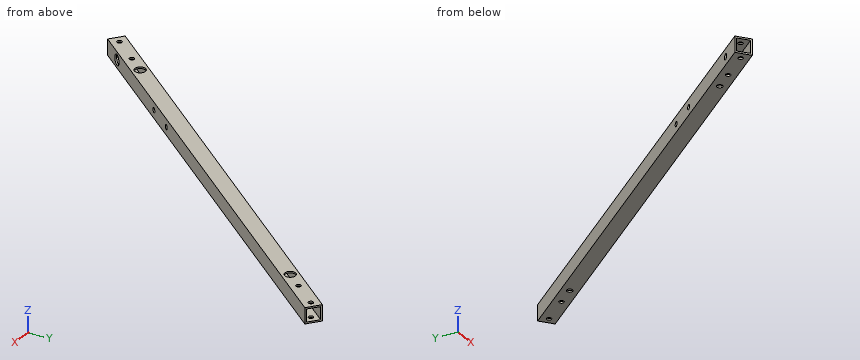
```python
from build123d import *

# Parameters (mm, degrees)
EXTRUDE_1_DEPTH             = 15
SHELL_1_T                   = -1.5
SKETCH_3_R                  = 2.25
SKETCH_3_R_2                = 2.7
CUT_EXTRUDE_1_DEPTH         = 25
SKETCH_5_R                  = 2.25
SKETCH_5_R_2                = 2.7
CUT_EXTRUDE_3_DEPTH         = 20
SKETCH_7_W                  = 15
SKETCH_7_H                  = 15
SKETCH_7_W_2                = 12
SKETCH_7_H_2                = 12
CUT_EXTRUDE_4_DEPTH         = 1
HOLE_WIZARD_10_0_10_1_D     = 10
HOLE_WIZARD_10_0_10_1_DEPTH = 1.5
HOLE_WIZARD_10_0_10_2_D     = 10
HOLE_WIZARD_10_0_10_2_DEPTH = 1.5


with BuildPart() as part:
    # ｽｹｯﾁ1 → ﾎﾞｽ - 押し出し1 (new body)
    with BuildSketch(Plane.XY):
        Polygon((306.8847856, 365.731045751), (0, 0), (-11.490666647, 9.641814145), (295.394118953, 375.372859896), align=None)
    extrude(amount=EXTRUDE_1_DEPTH)

    # ｼｪﾙ1
    shell_1_openings = [part.faces().sort_by_distance(p)[0] for p in [
        (301.139452276, 370.551952824, 7.5),
        (-5.745333323, 4.820907073, 7.5),
    ]]
    offset(amount=SHELL_1_T, openings=shell_1_openings, kind=Kind.INTERSECTION)

    # ｽｹｯﾁ3 → ｶｯﾄ - 押し出し1 (cut)
    with BuildSketch(Plane.XY.offset(15)):
        with Locations((-0.924426251, 10.566240396)):
            Circle(SKETCH_3_R)
        with Locations((18.35920204, 33.54757369)):
            Circle(SKETCH_3_R)
        with Locations((277.034916913, 341.825286207)):
            Circle(SKETCH_3_R)
        with Locations((296.318545204, 364.8066195)):
            Circle(SKETCH_3_R)
        with Locations((31.214954234, 48.868462552)):
            Circle(SKETCH_3_R_2)
        with Locations((264.179164719, 326.504397344)):
            Circle(SKETCH_3_R_2)
    extrude(amount=-CUT_EXTRUDE_1_DEPTH, mode=Mode.SUBTRACT)

    # ｽｹｯﾁ5 → ｶｯﾄ - 押し出し3 (cut)
    with BuildSketch(Plane(origin=(-11.490666647, 9.641814145, 0), x_dir=(0, 0, 1), z_dir=(-0.766044443, 0.64278761, 0))):
        with Locations((7.5, 141.822406051)):
            Circle(SKETCH_5_R)
        with Locations((7.5, 111.822406051)):
            Circle(SKETCH_5_R)
        with Locations((7.5, 22.5)):
            Circle(SKETCH_5_R_2)
    extrude(amount=-CUT_EXTRUDE_3_DEPTH, mode=Mode.SUBTRACT)

    # ｽｹｯﾁ7 → ｶｯﾄ - 押し出し4 (cut)
    with BuildSketch(Plane(origin=(306.8847856, 365.731045751, 0), x_dir=(0.766044443, -0.64278761, 0), z_dir=(0.64278761, 0.766044443, 0))):
        with Locations((-7.5, -7.5)):
            Rectangle(SKETCH_7_W, SKETCH_7_H)
        with Locations((-7.5, -7.5)):
            Rectangle(SKETCH_7_W_2, SKETCH_7_H_2, mode=Mode.SUBTRACT)
    extrude(amount=-CUT_EXTRUDE_4_DEPTH, mode=Mode.SUBTRACT)

    # Ø10.0 (10) 直径の穴1
    with Locations(Plane(origin=(0, 0, 0), x_dir=(0, 0, -1), z_dir=(0.766044443, -0.64278761, 0))):
        with Locations((-7.5, 22.5)):
            Hole(HOLE_WIZARD_10_0_10_1_D / 2, depth=HOLE_WIZARD_10_0_10_1_DEPTH)

    # Ø10.0 (10) 直径の穴2
    with Locations(Plane.XY.offset(15)):
        with Locations((31.214954234, 48.868462552), (264.179164719, 326.504397344)):
            Hole(HOLE_WIZARD_10_0_10_2_D / 2, depth=HOLE_WIZARD_10_0_10_2_DEPTH)


solid = part.part
```
Geometry check sheet. Reference: the model listing, model coordinates, mm. Give positions to 0.01 mm unless a question says otherwise; leave off trailing zeros. Order: outer loops, then holes, each group sorted by start corner. A loop starts at its lowest first (then second) coordinate and runs counter-clockwise, first axis right, second up. Notation, with made-up numbers: (33, -8) - (63, -8) arc R34 ccw to (63, 30) - close; hole circle Ø7 at (0.5, 71.5). An arc over 180 degrees is marked (long way). Write item = value, one per line. Start each with the question number.
1) Section check B-B (y = 249). Enter the section's corners in (x, z), then the cut area to 3 significant figures.
2) Scan lines: L1, parallel to Y at x = 191, z = 10.5; L2, parallel to Y at x = 83, z = 11.75; L3, parallel to X at y = 320.5, z = 3.25. Record each from-to range of solid material in increasing order.
3) Section check A-A (x = 151.5). Enter the section's corners in (y, z), then the cut area to 3 significant figures.
4) Gauge pin test, flat ends, axial feed: pin 1 Ø5 at (y, z) = (165, 2.5) entering from +X; pin 2 Ø1.5 at (y, z) = (79, 13.5) entering from +X; pin 3 Ø1 at (x, z) = (173.5, 2.5) entering from +Y. Record the tip position at first contact, or that the pin passes through.
Geometry check:
q1.outline = (189.35, 0) - (208.94, 0) - (208.94, 15) - (189.35, 15) - close; hole (191.31, 1.5) - (206.98, 1.5) - (206.98, 13.5) - (191.31, 13.5) - close
q1.area = 106 mm2
q2.L1 = 227.62 to 229.96, 248.63 to 250.96
q2.L2 = 98.92 to 101.25, 119.92 to 122.25
q2.L3 = 249.35 to 251.31, 266.97 to 268.93
q3.outline = (180.55, 0) - (203.89, 0) - (203.89, 15) - (180.55, 15) - close; hole (182.88, 1.5) - (201.55, 1.5) - (201.55, 13.5) - (182.88, 13.5) - close
q3.area = 126 mm2
q4.pin_1 = 140.55
q4.pin_2 = 66.92
q4.pin_3 = 230.7
